```python
from build123d import *

# Parameters (mm, degrees)
SKETCH1_W           = 228.6
SKETCH1_H           = 215.9
BOSS_EXTRUDE1_DEPTH = 6.35
SKETCH8_W           = 25.4
SKETCH8_H           = 6.35
CUT_EXTRUDE2_DEPTH  = 7.35
SKETCH11_R          = 1.524
CUT_EXTRUDE4_DEPTH  = 7.35
CUT_EXTRUDE5_DEPTH  = 7.35
BOSS_EXTRUDE3_DEPTH = 152.4


with BuildPart() as part:
    # Sketch1 → Boss-Extrude1 (new body)
    with BuildSketch(Plane(origin=(0, 0, 0), x_dir=(1, 0, 0), z_dir=(0, 1, 0))):
        with Locations((114.3, 107.95)):
            Rectangle(SKETCH1_W, SKETCH1_H)
    extrude(amount=BOSS_EXTRUDE1_DEPTH)

    # Sketch8 → Cut-Extrude2 (cut, through all)
    with BuildSketch(Plane(origin=(0, 6.35, 0), x_dir=(1, 0, 0), z_dir=(0, 1, 0))):
        with Locations((19.05, 132.334)):
            Rectangle(SKETCH8_W, SKETCH8_H)
        with Locations((209.55, 132.334)):
            Rectangle(SKETCH8_W, SKETCH8_H)
        with Locations((209.55, 83.566)):
            Rectangle(SKETCH8_W, SKETCH8_H)
        with Locations((19.05, 83.566)):
            Rectangle(SKETCH8_W, SKETCH8_H)
    extrude(amount=-CUT_EXTRUDE2_DEPTH, mode=Mode.SUBTRACT)

    # Sketch11 → Cut-Extrude4 (cut, through all)
    with BuildSketch(Plane(origin=(0, 6.35, 0), x_dir=(1, 0, 0), z_dir=(0, 1, 0))):
        with Locations((95.758, 6.604)):
            Circle(SKETCH11_R)
        with Locations((132.842, 6.604)):
            Circle(SKETCH11_R)
        with Locations((132.842, 43.688)):
            Circle(SKETCH11_R)
        with Locations((95.758, 43.688)):
            Circle(SKETCH11_R)
    extrude(amount=-CUT_EXTRUDE4_DEPTH, mode=Mode.SUBTRACT)

    # Sketch13 → Cut-Extrude5 (cut, through all)
    with BuildSketch(Plane(origin=(0, 6.35, 0), x_dir=(1, 0, 0), z_dir=(0, 1, 0))):
        Polygon((0, 215.9), (0, 161.925), (57.15, 215.9), align=None)
        Polygon((228.6, 161.925), (171.45, 215.9), (228.6, 215.9), align=None)
        Polygon((228.6, 0), (228.6, 53.975), (171.45, 0), align=None)
        Polygon((0, 53.975), (57.15, 0), (0, 0), align=None)
    extrude(amount=-CUT_EXTRUDE5_DEPTH, mode=Mode.SUBTRACT)

    # Sketch18 → Boss-Extrude3 (add)
    with BuildSketch(Plane(origin=(0, 6.35, 0), x_dir=(1, 0, 0), z_dir=(0, 1, 0))):
        Polygon((114.3, 166.095906935), (99.839700965, 164.269146346), (86.2879957, 158.903646664), (74.496387686, 150.336541968), (65.205787021, 139.106134954), (58.999956314, 125.918073396), (56.26883073, 111.601011705), (57.184016936, 97.054543521), (61.688010415, 83.192676938), (69.497808694, 70.886404014), (80.122693423, 60.908973136), (92.895064019, 53.887302981), (107.012385465, 50.262590909), (121.587614535, 50.262590909), (135.704935981, 53.887302981), (148.477306577, 60.908973136), (159.102191306, 70.886404014), (166.911989585, 83.192676938), (171.415983064, 97.054543521), (172.33116927, 111.601011705), (169.600043686, 125.918073396), (163.394212979, 139.106134954), (154.103612314, 150.336541968), (142.3120043, 158.903646664), (128.760299035, 164.269146346), align=None)
        Polygon((114.3, 162.56), (100.719045262, 160.844326429), (87.991431857, 155.805107797), (76.916882545, 147.758976743), (68.191251988, 137.211501274), (62.362803645, 124.825418063), (59.797760361, 111.378990271), (60.657293238, 97.71710641), (64.887394665, 84.698192888), (72.222271812, 73.14027592), (82.201047372, 63.769581937), (94.196718178, 57.174906106), (107.455552115, 53.770616161), (121.144447885, 53.770616161), (134.403281822, 57.174906106), (146.398952628, 63.769581937), (156.377728188, 73.14027592), (163.712605335, 84.698192888), (167.942706762, 97.71710641), (168.802239639, 111.378990271), (166.237196355, 124.825418063), (160.408748012, 137.211501274), (151.683117455, 147.758976743), (140.608568143, 155.805107797), (127.880954738, 160.844326429), align=None, mode=Mode.SUBTRACT)
    extrude(amount=BOSS_EXTRUDE3_DEPTH)


solid = part.part
```
Build history of the part. All positions in model axes, mm. A direction names the side the tool comes from. Round coordinates to 2 decimals unless told otherwise and drop trailing zeros. Write each loop counter-clockwise with the first axis right and the second up, starting at its lowest first coordinate (ties: lowest second). Pieces come first, ordered by that corner, then holes. Notation, with made-up numbers: (-38.75, 75.5) - (-25.75, 75.5) arc R16 ccw to (-25.75, 83.5) - close; hole circle Ø6 at (-23.75, 44.5). An arc over 180 degrees is marked (long way). Write each question's results on one line, items separated by ' | '. Start each with the question number.
Item 1: Saw through at D-D (z = -196). Write the cut outline in (x, y).
Item 2: Wall check: L1, parallel to X at y = 95, z = -110.5; L2, parallel to Y at x = 35, z = -67; L3, parallel to X at y = 43.5, z = -115. Give the ranges that are in metal, low to high. Write a range as [from, to].
Item 3: Saw through at B-B (z = -117). Write the cut outline in (x, y).
Item 4: Mould opens along Z. For faces 5 (the face through (158.814, 81.483, -144.643)), 6 (the face through (151.32, 81.48, -68.39)), 7 (the face through (153.72, 81.48, -65.83)) say: pulls with the +Z half, pulls with the -Z half, needs draft (parallel to the pull), parting line crosses it, or undercut.
Item 5: Saw through at C-C (x = 24). Write the cut outline in (y, z), and give its area (3 significant figures).
Item 6: Drop flat-ended pins along their axis: P1, Ø3, axis at x = 156.5, y = 82, coming from the +Z side; P2, Ø3, axis at x = 23.5, y = 2.5, coming from the -Z side; P3, Ø5, axis at x = 207.5, y = 4, coming from the -Z side. Give the stop position or say it passes through.
Item 7: Saw through at A-A (x = 211.5). Write the cut outline in (y, z) (3 decimals).
Item 8: Which spindle directions (+Z, -Z, +X, -X, +Y, -Y) get a long thin tool onto all of the face, cutting with end or side? Do faces 1 (the face through (62.146, 81.483, -132.604)), 2 (the face through (121.63, 81.48, -165.17)), 3 (the face through (65.32, 81.48, -131.11)), 4 (the face through (19, 3, -86.741)). Say none if no direction does.
Results are:
1) outline: (36.08, 0) - (192.52, 0) - (192.52, 6.35) - (36.08, 6.35) - close
2) L1: x = [56.34, 59.85], [168.75, 172.26] | L2: y = [0, 6.35] | L3: x = [56.92, 60.49], [168.11, 171.68]
3) outline: (0, 0) - (228.6, 0) - (228.6, 6.35) - (171.3, 6.35) - (171.3, 158.75) - (167.73, 158.75) - (167.73, 6.35) - (60.87, 6.35) - (60.87, 158.75) - (57.3, 158.75) - (57.3, 6.35) - (0, 6.35) - close
4) face 5: pulls with the -Z half | face 6: undercut | face 7: pulls with the +Z half
5) outline: (0, -184.59) - (6.35, -184.59) - (6.35, -135.51) - (0, -135.51) - close; (0, -129.16) - (6.35, -129.16) - (6.35, -86.74) - (0, -86.74) - close; (0, -80.39) - (6.35, -80.39) - (6.35, -31.31) - (0, -31.31) - close | area: 893 mm²
6) P1: stops at z = -67.03 | P2: stops at z = -185.54 | P3: stops at z = -184.21
7) outline: (0, -178.075) - (6.35, -178.075) - (6.35, -135.509) - (0, -135.509) - close; (0, -129.159) - (6.35, -129.159) - (6.35, -86.741) - (0, -86.741) - close; (0, -80.391) - (6.35, -80.391) - (6.35, -37.825) - (0, -37.825) - close
8) face 1: -Z, -X, +Y | face 2: -Z, +X, +Y | face 3: +Y | face 4: +Y, -Y
